```python
from build123d import *

# Parameters (mm, degrees)
BOSS_EXTRUDE1_DEPTH     = 50
CUT_EXTRUDE1_DEPTH      = 731.807873314
CUT_EXTRUDE1_DEPTH_BACK = 731.807873314
SKETCH2_R               = 10


with BuildPart() as part:
    # Sketch1 → Boss-Extrude1 (new body)
    with BuildSketch(Plane(origin=(0, 0, 0), x_dir=(1, 0, 0), z_dir=(0, 1, 0))):
        Polygon((-424.861111111, 294.975010995), (273.138888889, 294.975010995), (273.138888889, 93.975010995), (374.138888889, 93.975010995), (374.138888889, -304.024989005), (269.138888889, -304.024989005), (269.138888889, -505.024989005), (-424.861111111, -505.024989005), (-424.861111111, -304.024989005), (-525.861111111, -304.024989005), (-525.861111111, 93.975010995), (-424.861111111, 93.975010995), align=None)
    extrude(amount=BOSS_EXTRUDE1_DEPTH)

    # Sketch2 → Cut-Extrude1 (cut, two sides: drawn at the far end of the back side and taken through both)
    with BuildSketch(Plane(origin=(0, 50, 0), x_dir=(1, 0, 0), z_dir=(0, 1, 0)).offset(-CUT_EXTRUDE1_DEPTH_BACK)):
        Polygon((220.982294355, -35.192293353), (220.982294355, 3.725435945), (220.982294355, 74.807706647), (130.982294355, 74.807706647), (130.982294355, -5.192293353), (130.982294355, -35.192293353), align=None)
        with Locations(Location((175.982294355, -425.024989005, 0), (0, 0, 90))):
            Circle(SKETCH2_R)
        with Locations(Location((175.982294355, -169.024989005, 0), (0, 0, 90))):
            Circle(SKETCH2_R)
    extrude(amount=CUT_EXTRUDE1_DEPTH + CUT_EXTRUDE1_DEPTH_BACK, mode=Mode.SUBTRACT)


solid = part.part
```
For this review, take the finished solid that the model builds, in its own axes (mm). A direction names the side the tool comes from. Coordinates: 2 decimals unless noted, no trailing zeros. Write each loop counter-clockwise with the first axis right and the second up, starting at its lowest first coordinate (ties: lowest second). Pieces come first, ordered by that corner, then holes. Notation, with made-up numbers: (-20.5, 31.25) -> (29.5, 31.25) arc R12 ccw to (29.5, 41.25) -> close; hole circle Ø2 at (-21, 48). An arc over 180 degrees is marked (long way). Put each result on its own line as item: value.
Q1. The part is to be moulded in two halves that separate along X. For faces 1 (the flat face through (177, 25, -74.808)), 2 (the flat face through (-424.861, 25, -193)), 3 (the flat face through (273.139, 25, -196)), say which applies: +X half, -X half, draft (parallel to the pull), parting line (faces both ways), or undercut.
From the geometry:
face 1: undercut
face 2: -X half
face 3: +X half
Q2. Take a section at C-C, the plane z = 330.5. State the section outline as (x, y) points, then the cut area to 3 significant figures.
From the geometry:
outline: (-424.86, 0) -> (269.14, 0) -> (269.14, 50) -> (-424.86, 50) -> close
area: 34,700 mm2
Q3. Clearance check with flat-ended pins moving along their axes: pin 1 Ø25 at (y, z) = (33.5, 375.5) entering from -X; pin 2 Ø15 at (y, z) = (26.5, -165) entering from +X; pin 3 Ø25 at (x, y) = (296.5, 24) entering from +Z (3 decimals). State where each tip first meets the part, or that it passes through.
From the geometry:
pin 1: stops at x = -424.86
pin 2: stops at x = 273.14
pin 3: stops at z = 304.025
Q4. Tool access review of faces 4 (the flat face through (323, 25, -93.975)), 5 (the flat face through (-476, 25, -93.975)), 6 (the flat face through (130.982, 25, -21)): name each direction out of +Z, -Z, +X, -X, +Y, -Y from which nothing blocks a thin tool from reaching the whole face with its end or side.
From the geometry:
face 4: -Z, +X, +Y, -Y
face 5: -Z, -X, +Y, -Y
face 6: +Y, -Y
Q5. Take a section at D-D, the plane x = -464. State the section outline as (y, z) points, then the cut area to 3 significant figures.
From the geometry:
outline: (0, -93.98) -> (50, -93.98) -> (50, 304.02) -> (0, 304.02) -> close
area: 19,900 mm2
Q6. Take a section at A-A, the plane z = 21. State the section outline as (x, y) points, then the cut area to 3 significant figures.
From the geometry:
outline: (-525.86, 0) -> (130.98, 0) -> (130.98, 50) -> (-525.86, 50) -> close; (220.98, 0) -> (374.14, 0) -> (374.14, 50) -> (220.98, 50) -> close
area: 40,500 mm2
Q7. Wall thickness on L1, parallel to Z at x = 159, y = 6; L2, parallel to Z at x = 184, y = 37.5; L3, parallel to X at y = 13, z = -40.5: over which ranges is each line inside the solid? List them lowest first.
From the geometry:
L1: z = -294.98 to -74.81, 35.19 to 505.02
L2: z = -294.98 to -74.81, 35.19 to 163.05, 175 to 419.05, 431 to 505.02
L3: x = -525.86 to 130.98, 220.98 to 374.14
Q8. Take a section at B-B, the plane y = 15. State the section outline as (x, z) points.
From the geometry:
outline: (-525.86, -93.98) -> (-424.86, -93.98) -> (-424.86, -294.98) -> (273.14, -294.98) -> (273.14, -93.98) -> (374.14, -93.98) -> (374.14, 304.02) -> (269.14, 304.02) -> (269.14, 505.02) -> (-424.86, 505.02) -> (-424.86, 304.02) -> (-525.86, 304.02) -> close; hole (130.98, -74.81) -> (220.98, -74.81) -> (220.98, 35.19) -> (130.98, 35.19) -> close; hole circle Ø20 at (175.98, 169.02); hole circle Ø20 at (175.98, 425.02)
